The model under review builds one solid part; all positions refer to its coordinate system, in mm. Face numbers are marked on the shaded views. A direction names the side the tool comes from. Round coordinates to 2 decimals unless told otherwise and drop trailing zeros. Write each loop counter-clockwise with the first axis right and the second up, starting at its lowest first coordinate (ties: lowest second). Pieces come first, ordered by that corner, then holes. Notation, with made-up numbers: (77, -3.5) -> (103, -3.5) arc R20 ccw to (103, 35.5) -> close; hole circle Ø5 at (40, -22). An arc over 180 degrees is marked (long way). Use CSV: the item, a comma, the result in double quotes. Start each with the question number.
1) Take a section at C-C, the plane x = 21. Give the boundary of the cut face in (y, z).
2) Take a section at B-B, the plane y = 2.75. Give the boundary of the cut face in (x, z).
3) Machinability: for the marked faces 1 and 2, which of the approach directions +Z, -Z, +X, -X, +Y, -Y give a long, thin tool a straight path to every point of the face, cutting with its end or side? Answer none if there is none.
4) For pin 1 Ø14.5 at (x, z) = (16, 0) entering from +Y; pin 2 Ø4 at (x, y) = (13.5, 4.5) entering from -Z; pin 3 Ø3 at (x, y) = (9.5, 4) entering from +Z; pin 4 Ø3 at (y, z) = (1.5, 7) entering from -X (3 decimals), all flat-tipped, find the tip position at first contact; note any pin that passes through.
5) Take a section at D-D, the plane x = 29. Give the boundary of the cut face in (y, z).
6) Take a section at A-A, the plane x = 16. Give the boundary of the cut face in (y, z), then the cut area to 3 significant figures.
7) Wall thickness on probe 1 along X at (y, z) = (2, -21.5); probe 2 along Z at (x, y) = (16, 4.25); probe 3 along X at (y, z) = (1.5, -6): over which ranges is each line inside the solid? List them lowest first. Write a range as [from, to].
8) Mouldability with a two-part tool opening along X and no side actions: class the marked faces 3, 4 and 5 as released by +X, released by -X, zero draft, split by the parting line, or undercut.
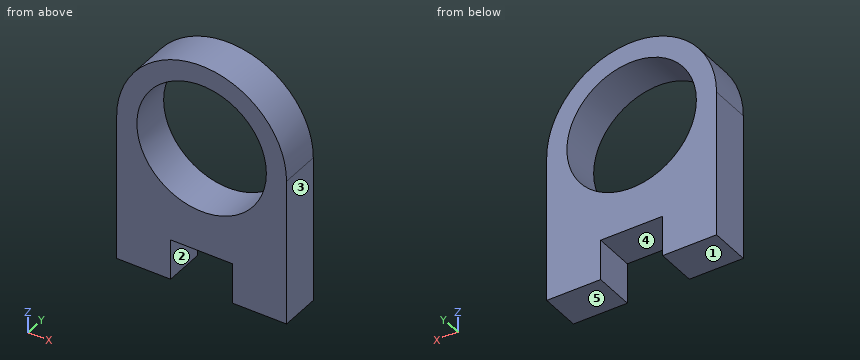
from build123d import *

# Parameters (mm, degrees)
BOSS_EXTRUDE1_DEPTH = 7.62
SKETCH2_R           = 12.2
CUT_EXTRUDE1_DEPTH  = 8.62
SKETCH3_W           = 10.16
SKETCH3_H           = 7.62
BOSS_EXTRUDE2_DEPTH = 7.62


with BuildPart() as part:
    # Sketch1 → Boss-Extrude1 (new body)
    with BuildSketch(Plane(origin=(0, 0, 0), x_dir=(1, 0, 0), z_dir=(0, 1, 0))):
        with BuildLine():
            Line((0, 0), (0, 20))
            Line((0, 20), (32, 20))
            Line((32, 20), (32, 0))
            ThreePointArc((32, 0), (16, -16), (0, 0))
        make_face()
    extrude(amount=BOSS_EXTRUDE1_DEPTH)

    # Sketch2 → Cut-Extrude1 (cut, through all)
    with BuildSketch(Plane.XZ):
        with Locations((16, 0)):
            Circle(SKETCH2_R)
    extrude(amount=-CUT_EXTRUDE1_DEPTH, mode=Mode.SUBTRACT)

    # Sketch3 → Boss-Extrude2 (add)
    with BuildSketch(Plane(origin=(0, 0, -20), x_dir=(-1, 0, 0), z_dir=(0, 0, -1))):
        with Locations((-26.92, 3.81)):
            Rectangle(SKETCH3_W, SKETCH3_H)
        with Locations((-5.08, 3.81)):
            Rectangle(SKETCH3_W, SKETCH3_H)
    extrude(amount=BOSS_EXTRUDE2_DEPTH)


solid = part.part
Values found:
1,outline,"(0, -20) -> (7.62, -20) -> (7.62, -11.13) -> (0, -11.13) -> close; (0, 11.13) -> (7.62, 11.13) -> (7.62, 15.2) -> (0, 15.2) -> close"
2,outline,"(0, -27.62) -> (10.16, -27.62) -> (10.16, -20) -> (21.84, -20) -> (21.84, -27.62) -> (32, -27.62) -> (32, 0) arc R16 ccw to (0, 0) -> close; hole circle Ø24.4 at (16, 0)"
3,face 1,"-Z, +X, -X, +Y, -Y"
3,face 2,"-Z, +Y, -Y"
4,pin 1,"through"
4,pin 2,"z = -20"
4,pin 3,"z = 15.2"
4,pin 4,"x = 0.975"
5,outline,"(0, -27.62) -> (7.62, -27.62) -> (7.62, 9.33) -> (0, 9.33) -> close"
6,outline,"(0, -20) -> (7.62, -20) -> (7.62, -12.2) -> (0, -12.2) -> close; (0, 12.2) -> (7.62, 12.2) -> (7.62, 16) -> (0, 16) -> close"
6,area,"88.4 mm²"
7,probe 1,"[0, 10.16], [21.84, 32]"
7,probe 2,"[-20, -12.2], [12.2, 16]"
7,probe 3,"[0, 5.38], [26.62, 32]"
8,face 3,"released by +X"
8,face 4,"undercut"
8,face 5,"zero draft"
